```python
from build123d import *

# Parameters (mm, degrees)
SKETCH1_W            = 326.5
SKETCH1_H            = 82
BOSS_EXTRUDE1_DEPTH  = 1.5875
SKETCH2_R            = 10
CUT_EXTRUDE1_DEPTH   = 337.643387216
FILLET1_R            = 5
FILLET2_R            = 5
FILLET1_OF_MIRROR1_R = 5
FILLET2_OF_MIRROR1_R = 5


with BuildPart() as part:
    # Sketch1 → Boss-Extrude1 (new body)
    with BuildSketch(Plane.XY):
        with Locations((163.25, -41)):
            Rectangle(SKETCH1_W, SKETCH1_H)
    extrude(amount=BOSS_EXTRUDE1_DEPTH)

    # Sketch2 → Cut-Extrude1 (cut, through all)
    with BuildSketch(Plane.XY.offset(1.5875)):
        with BuildLine():
            Line((261.25, -60.453756551), (261.25, -21.546243449))
            ThreePointArc((261.25, -21.546243449), (258.421566961, -17.042434291), (253.136281226, -17.634114183))
            Line((253.136281226, -17.634114183), (231.985399239, -34.468399005))
            ThreePointArc((231.985399239, -34.468399005), (233.246092528, -40.630207826), (232.246877073, -46.839781402))
            Line((232.246877073, -46.839781402), (253.036061952, -64.283978766))
            ThreePointArc((253.036061952, -64.283978766), (258.363091309, -64.985295486), (261.25, -60.453756551))
        make_face()
        with BuildLine():
            ThreePointArc((205.742038309, -26.644140472), (215.75, -23.5), (225.757961691, -26.644140472))
            Line((225.757961691, -26.644140472), (241.754677282, -13.912129266))
            ThreePointArc((241.754677282, -13.912129266), (243.361162229, -8.350855727), (238.640958508, -5))
            Line((238.640958508, -5), (192.859041492, -5))
            ThreePointArc((192.859041492, -5), (188.138837771, -8.350855727), (189.745322718, -13.912129266))
            Line((189.745322718, -13.912129266), (205.742038309, -26.644140472))
        make_face()
        with BuildLine():
            Line((241.754677282, -68.087870734), (225.757961691, -55.355859528))
            ThreePointArc((225.757961691, -55.355859528), (215.75, -58.5), (205.742038309, -55.355859528))
            Line((205.742038309, -55.355859528), (189.745322718, -68.087870734))
            ThreePointArc((189.745322718, -68.087870734), (188.138837771, -73.649144273), (192.859041492, -77))
            Line((192.859041492, -77), (238.640958508, -77))
            ThreePointArc((238.640958508, -77), (243.361162229, -73.649144273), (241.754677282, -68.087870734))
        make_face()
        with BuildLine():
            ThreePointArc((199.253122927, -46.839781402), (198.253907472, -40.630207826), (199.514600761, -34.468399005))
            Line((199.514600761, -34.468399005), (178.363718774, -17.634114183))
            ThreePointArc((178.363718774, -17.634114183), (173.078433039, -17.042434291), (170.25, -21.546243449))
            Line((170.25, -21.546243449), (170.25, -60.453756551))
            ThreePointArc((170.25, -60.453756551), (173.136908691, -64.985295486), (178.463938048, -64.283978766))
            Line((178.463938048, -64.283978766), (199.253122927, -46.839781402))
        make_face()
        with BuildLine():
            Line((313, -5), (293.910254038, -5))
            ThreePointArc((293.910254038, -5), (289.080624906, -8.705904774), (291.410254038, -14.330127019))
            Line((291.410254038, -14.330127019), (310.5, -25.351596989))
            ThreePointArc((310.5, -25.351596989), (315.5, -25.351596989), (318, -21.02146997))
            Line((318, -21.02146997), (318, -10))
            ThreePointArc((318, -10), (316.535533906, -6.464466094), (313, -5))
        make_face()
        with BuildLine():
            ThreePointArc((315.5, -42.214646281), (316.262390864, -41.673556851), (316.910726246, -41))
            ThreePointArc((316.910726246, -41), (316.262390864, -40.326443149), (315.5, -39.785353719))
            Line((315.5, -39.785353719), (282.75, -20.877132403))
            ThreePointArc((282.75, -20.877132403), (277.75, -20.877132403), (275.25, -25.207259422))
            Line((275.25, -25.207259422), (275.25, -56.792740578))
            ThreePointArc((275.25, -56.792740578), (277.75, -61.122867597), (282.75, -61.122867597))
            Line((282.75, -61.122867597), (315.5, -42.214646281))
        make_face()
        with BuildLine():
            Line((310.5, -56.648403011), (291.410254038, -67.669872981))
            ThreePointArc((291.410254038, -67.669872981), (289.080624906, -73.294095226), (293.910254038, -77))
            Line((293.910254038, -77), (313, -77))
            ThreePointArc((313, -77), (316.535533906, -75.535533906), (318, -72))
            Line((318, -72), (318, -60.97853003))
            ThreePointArc((318, -60.97853003), (315.5, -56.648403011), (310.5, -56.648403011))
        make_face()
        with Locations((215.75, -41)):
            Circle(SKETCH2_R)
    cut_extrude1 = extrude(amount=-CUT_EXTRUDE1_DEPTH, mode=Mode.SUBTRACT)

    # Fillet1
    fillet1_edges = [part.edges().sort_by_distance(p)[0] for p in [
        (232.246877073, -46.839781402, 0.79375),
        (231.985399239, -34.468399005, 0.79375),
        (205.742038309, -55.355859528, 0.79375),
        (225.757961691, -55.355859528, 0.79375),
        (199.514600761, -34.468399005, 0.79375),
        (199.253122927, -46.839781402, 0.79375),
        (225.757961691, -26.644140472, 0.79375),
        (205.742038309, -26.644140472, 0.79375),
    ]]
    fillet(fillet1_edges, radius=FILLET1_R)

    # Fillet2
    fillet2_edges = [part.edges().sort_by_distance(p)[0] for p in [
        (316.910726246, -41, 0.79375),
    ]]
    fillet(fillet2_edges, radius=FILLET2_R)

    # Mirror1: Cut-Extrude1 across plane
    add(cut_extrude1.mirror(Plane.ZY.offset(-163.25)), mode=Mode.SUBTRACT)

    # Fillet1 of Mirror1
    fillet1_of_mirror1_edges = [part.edges().sort_by_distance(p)[0] for p in [
        (94.253122927, -46.839781402, 0.79375),
        (94.514600761, -34.468399005, 0.79375),
        (120.757961691, -55.355859528, 0.79375),
        (100.742038309, -55.355859528, 0.79375),
        (126.985399239, -34.468399005, 0.79375),
        (127.246877073, -46.839781402, 0.79375),
        (100.742038309, -26.644140472, 0.79375),
        (120.757961691, -26.644140472, 0.79375),
    ]]
    fillet(fillet1_of_mirror1_edges, radius=FILLET1_OF_MIRROR1_R)

    # Fillet2 of Mirror1
    fillet2_of_mirror1_edges = [part.edges().sort_by_distance(p)[0] for p in [
        (9.589273754, -41, 0.79375),
    ]]
    fillet(fillet2_of_mirror1_edges, radius=FILLET2_OF_MIRROR1_R)


solid = part.part
```
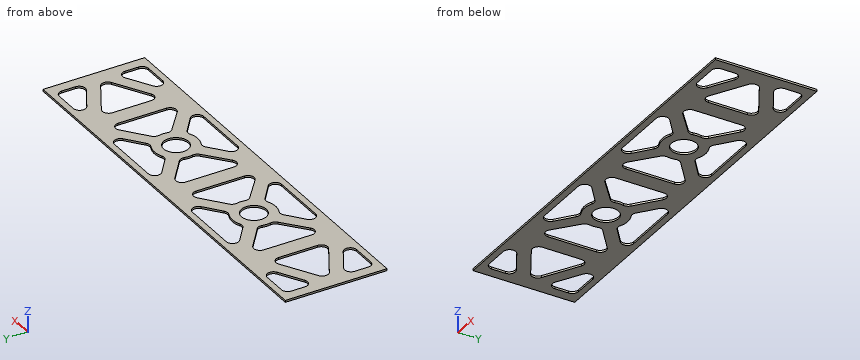
Design review of the part built by this model. Coordinates are the model's own, in mm. Coordinates: 2 decimals unless noted, no trailing zeros. Order: outer loops, then holes, each group sorted by start corner. A loop starts at its lowest first (then second) coordinate and runs counter-clockwise, first axis right, second up. Notation, with made-up numbers: (81.25, 62.25) -> (133.25, 62.25) arc R24 ccw to (133.25, 74.25) -> close; hole circle Ø4 at (66, 14.5). An arc over 180 degrees is marked (long way). One line per item, written item: value. Start each with the question number.
Q1. Take a section at A-A, the plane x = 110.75. State the section outline as (y, z) points.
Q2. For probe 1 along Y at (x, z) = (175, 0.1); probe 2 along X at (y, z) = (-70.5, 0.85); probe 3 along Y at (x, z) = (26, 0.25), list the stretches that pass through material, from the lowest coordinate up.
Q3. Take a section at B-B, the plane y = -41. Give the number of separate pieces and of enclosed holes in the cut face, then the cut area to 3 significant figures.
Q4. Take a section at D-D, the plane x = 21. State the section outline as (y, z) points.
Q5. Insertion check: pin 1 Ø0.8 at (x, z) = (227, 1) entering from +Y; pin 2 Ø16 at (x, y) = (110.75, -41) entering from -Z. Each pin has a flat end and moves straight along its axis. Give the tip position at first contact, or say it passes through.
Values follow:
1. outline: (-82, 0) -> (-77, 0) -> (-77, 1.59) -> (-82, 1.59) -> close; (-58.5, 0) -> (-51, 0) -> (-51, 1.59) -> (-58.5, 1.59) -> close; (-31, 0) -> (-23.5, 0) -> (-23.5, 1.59) -> (-31, 1.59) -> close; (-5, 0) -> (0, 0) -> (0, 1.59) -> (-5, 1.59) -> close
2. probe 1: y = -82 to -65.45, -16.55 to 0
2. probe 2: x = 0 to 8.5, 37.36 to 83.09, 138.41 to 188.09, 243.41 to 289.14, 318 to 326.5
2. probe 3: y = -82 to -77, -62.42 to -50.87, -31.13 to -19.58, -5 to 0
3. separate pieces: 9
3. enclosed holes: 0
3. area: 158 mm2
4. outline: (-82, 0) -> (-77, 0) -> (-77, 1.59) -> (-82, 1.59) -> close; (-59.54, 0) -> (-47.99, 0) -> (-47.99, 1.59) -> (-59.54, 1.59) -> close; (-34.01, 0) -> (-22.46, 0) -> (-22.46, 1.59) -> (-34.01, 1.59) -> close; (-5, 0) -> (0, 0) -> (0, 1.59) -> (-5, 1.59) -> close
5. pin 1: stops at y = 0
5. pin 2: passes through
